Read the model definition and answer for the solid it produces. Units are mm, in the model's axes. Round coordinates to 2 decimals unless told otherwise and drop trailing zeros. Loops run counter-clockwise (first coordinate to the right, second up) from the corner with the lowest first, then second, coordinate; pieces in that order, holes last. Notation, with made-up numbers: (-20.5, 52) -> (21.5, 52) arc R20 ccw to (21.5, 62) -> close; hole circle Ø8 at (15, 71). An arc over 180 degrees is marked (long way). Put each result on its own line as item: value.
from build123d import *

# Parameters (mm, degrees)
SKETCH1_R           = 3.81
BOSS_EXTRUDE1_DEPTH = 2.54
BOSS_EXTRUDE2_DEPTH = 12.7


with BuildPart() as part:
    # Sketch1 → Boss-Extrude1 (new body)
    with BuildSketch(Plane.XY):
        Circle(SKETCH1_R)
        with BuildLine():
            Line((-0.933255592, 2.19075), (0.933255592, 2.19075))
            ThreePointArc((0.933255592, 2.19075), (0, -2.38125), (-0.933255592, 2.19075))
        make_face(mode=Mode.SUBTRACT)
    extrude(amount=BOSS_EXTRUDE1_DEPTH)

    # Sketch2 → Boss-Extrude2 (add)
    with BuildSketch(Plane(origin=(0, 0, 0), x_dir=(-1, 0, 0), z_dir=(0, 0, -1))):
        with BuildLine():
            Line((-0.933255592, 2.19075), (0.933255592, 2.19075))
            ThreePointArc((0.933255592, 2.19075), (0, 2.38125), (-0.933255592, 2.19075))
        make_face()
    extrude(amount=BOSS_EXTRUDE2_DEPTH)


solid = part.part
Item 1: Find the intervals of material crossed by line 1 along Y through (x, z) = (0, 0.7); line 2 along Z through (x, y) = (1, -2.25); line 3 along Y through (x, z) = (2, 0.5), in increasing order.
Derived:
line 1: y = -3.81 to -2.38, 2.19 to 3.81
line 2: z = 0 to 2.54
line 3: y = -3.24 to -1.29, 1.29 to 3.24
Item 2: For a pull along Y with two mould halves and no side action, classify faces 1 (the cylindrical face through (-0.83, -3.72, 1.25)), 2 (the flat face through (0, 2.191, -5)), 3 (the cylindrical face through (0.09, -2.38, 1.25)), 4 (the flat face through (-2, -2, 2.54)) as pulls with the +Y half, pulls with the -Y half, needs draft (parallel to the pull), parting line crosses it, or undercut.
Derived:
face 1: parting line crosses it
face 2: undercut
face 3: undercut
face 4: needs draft
Item 3: The part is cut by section A-A (y = 0). Determine the outline of the cut face in (x, z).
Derived:
outline: (-3.81, 0) -> (-2.38, 0) -> (-2.38, 2.54) -> (-3.81, 2.54) -> close; (2.38, 0) -> (3.81, 0) -> (3.81, 2.54) -> (2.38, 2.54) -> close
Item 4: The part is cut by section B-B (x = 0.25). Determine the outline of the cut face in (y, z), then the cut area to 3 significant figures.
Derived:
outline: (-3.8, 0) -> (-2.37, 0) -> (-2.37, 2.54) -> (-3.8, 2.54) -> close; (2.19, -12.7) -> (2.37, -12.7) -> (2.37, 0) -> (3.8, 0) -> (3.8, 2.54) -> (2.19, 2.54) -> close
area: 9.99 mm^2
Item 5: The part is cut by section C-C (y = 1.25). Determine the outline of the cut face in (x, z), then the cut area to 3 significant figures.
Derived:
outline: (-3.6, 0) -> (-2.03, 0) -> (-2.03, 2.54) -> (-3.6, 2.54) -> close; (2.03, 0) -> (3.6, 0) -> (3.6, 2.54) -> (2.03, 2.54) -> close
area: 7.99 mm^2
Item 6: The part is cut by section D-D (z = -4). Determine the outline of the cut face in (x, y), then the cut area to 3 significant figures.
Derived:
outline: (-0.93, 2.19) -> (0.93, 2.19) arc R2.38 ccw to start
area: 0.239 mm^2
Item 7: Flat-ended cylindrical pins translate along their axes: pin 1 Ø3 at (x, z) = (2, -11) entering from -Y; pin 2 Ø4 at (x, y) = (1.5, -1) entering from -Z. Find the tip coordinate at first contact, or state that the pin passes through.
Derived:
pin 1: stops at y = 2.19
pin 2: stops at z = 0
